Autodesk Inventor part; units mm, degrees
ref_plane "YZ Plane" through (0, 0, 0) normal (1, 0, 0) x (0, 1, 0)
ref_plane "XZ Plane" through (0, 0, 0) normal (0, 1, 0) x (-1, 0, 0)
ref_plane "XY Plane" through (0, 0, 0) normal (0, 0, 1) x (1, 0, 0)
sketch "Sketch1" plane through (0, 0, 0) normal (0, 0, 1) x (1, 0, 0)
  line L0 (0, 0) -> (0, -38.1)
  line L1 (0, -38.1) -> (1219.2, -38.1)
  line L2 (1219.2, 0) -> (1219.2, -38.1)
  line L3 (0, 0) -> (1219.2, 0)
  line L4 (0, 0) -> (914.4, 0)
  line L5 (914.4, 609.6) -> (0, 0)
  line L6 (914.4, 609.6) -> (1219.2, 0)
  line L7 (1219.2, 0) -> (1126.19, 0)
  line L8 (1119.8068, 0) -> (879.9218, 479.77)
  line L9 (1119.8068, 0) -> (1219.2, 0)
  line L10 (160.2668, 0) -> (879.9218, 479.77)
  dimension "d3" = 88.9
extrude "Extrusion1" add sketch "Sketch1" against normal blind 38.1 contours L5 L6 L3 L8 L10
properties part number "side1"
Part model, mm, in its own coordinate system. A direction names the side the tool comes from. Round coordinates to 2 decimals unless told otherwise and drop trailing zeros. Write each loop counter-clockwise with the first axis right and the second up, starting at its lowest first coordinate (ties: lowest second). Pieces come first, ordered by that corner, then holes. Notation, with made-up numbers: M -13,11 L 39,11 A13 cw 39,30 Z; hole C 6,-10.5 d6. An arc over 180 degrees is marked long. One line per question, with ' | ' between items.
(1) Saw through at D-D on x = 822. Write the cut outline in (y, z), then the cut area to 3 significant figures.
Answer key:
outline: M 441.16,-38.1 L 548,-38.1 L 548,0 L 441.16,0 Z | area: 4,070 mm^2
(2) Saw through at C-C on y = 495. Write the cut outline in (x, z), then the cut area to 3 significant figures.
Answer key:
outline: M 742.5,-38.1 L 971.7,-38.1 L 971.7,0 L 742.5,0 Z | area: 8,730 mm^2
(3) Saw through at B-B on z = -29. Write the cut outline in (x, y), then the cut area to 3 significant figures.
Answer key:
outline: M 0,0 L 160.27,0 L 879.92,479.77 L 1119.81,0 L 1219.2,0 L 914.4,609.6 Z | area: 141,000 mm^2
(4) Saw through at A-A on y = 308. Write the cut outline in (x, z).
Answer key:
outline: M 462,-38.1 L 622.27,-38.1 L 622.27,0 L 462,0 Z; M 965.81,-38.1 L 1065.2,-38.1 L 1065.2,0 L 965.81,0 Z
(5) Probe line 1 along X through (y, z) = (150, -8); line 2 along X through (y, z) = (86, -5); line 3 along X through (y, z) = (574, -25). List the from-to ranges inside material, lowest first.
Answer key:
line 1: x = 225 to 385.27, 1044.81 to 1144.2 | line 2: x = 129 to 289.27, 1076.81 to 1176.2 | line 3: x = 861 to 932.2
(6) Pin check, flat tips, straight feed: pin 1 (10 mm diameter, centred on x = 499, z = -16, fed in from +Y); pin 2 (1 mm diameter, centred on y = 545.5, z = -15.5, fed in from -X); pin 3 (4 mm diameter, centred on x = 1059.5, z = -20, fed in from -Y). Stop position of each tip, or through.
Answer key:
pin 1: stops at y = 336 | pin 2: stops at x = 817.5 | pin 3: stops at y = 116.61
(7) 3-axis set-ups, long thin cutter, end or side, ignore diameter. For faces 1 (the face through (463.601, 309.067, -18.783)), 2 (the face through (515.06, 236.53, -18.78)): which of +Z, -Z, +X, -X, +Y, -Y reach the whole face in a straight line?
Answer key:
face 1: +Z, -Z, -X, +Y | face 2: +Z, -Z, -Y
